The drawing under review shows one solid part. Ordinate dimensions are in mm from its lowest x, y, z. A direction names the side the tool comes from. Give positions to 0.01 mm unless a question says otherwise; leave off trailing zeros. Order: outer loops, then holes, each group sorted by start corner. A loop starts at its lowest first (then second) coordinate and runs counter-clockwise, first axis right, second up. Notation, with made-up numbers: (10, 32) -> (67, 32) arc R24 cw to (67, 71) -> close; hole circle Ø2 at (36.5, 81.5). An arc over 180 degrees is marked (long way). Return JSON: item names as keys, results as strings. Group by question number.
1) Add section B-B (y = 18.5). Give the boundary of the cut face in (x, z), then the cut area to 3 significant figures.
2) Add section C-C (z = 29.5). Give the boundary of the cut face in (x, y).
3) Add section A-A (x = 18). Give the boundary of the cut face in (y, z) (1 decimal), then the cut area to 3 significant figures.
4) Insertion check: P1, Ø2.5, axis at x = 22.5, y = 37, coming from the +Z side; P2, Ø5, axis at y = 38, z = 33.5, coming from the -X side (1 decimal); P3, Ø5, axis at x = 10, y = 24.5, coming from the -Z side. Each pin has a flat end and moves straight along its axis. Give the tip position at first contact, or say it passes through.
5) Add section D-D (x = 36.5). Give the boundary of the cut face in (y, z), then the cut area to 3 significant figures.
6) For the marked faces 1, 2 and 3, list the 3-axis set-ups (+Z, -Z, +X, -X, +Y, -Y) from which the entire face can be reached by the end or side of a thin tool; tool diameter is ignored.
7) To check wall thickness, follow line 1 along Y through (x, z) = (22.5, 13.2); line 2 along Y through (x, z) = (22, 14) (1 decimal); line 3 along Z through (x, y) = (4.5, 22). State the ranges of each line that lie inside material, in increasing order.
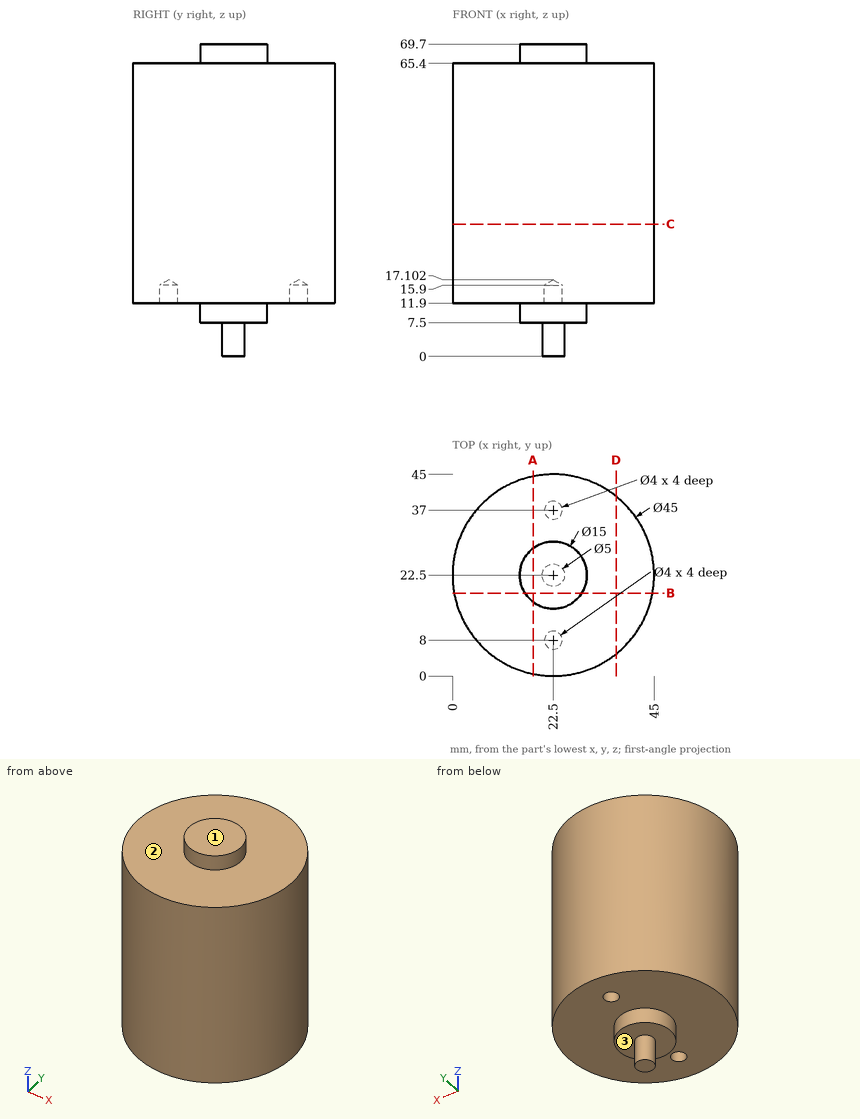
Evaluation:
{
 "1": {"outline": "(0.36, 11.9) -> (16.16, 11.9) -> (16.16, 7.5) -> (28.84, 7.5) -> (28.84, 11.9) -> (44.64, 11.9) -> (44.64, 65.4) -> (28.84, 65.4) -> (28.84, 69.7) -> (16.16, 69.7) -> (16.16, 65.4) -> (0.36, 65.4) -> close", "area": "2,480 mm^2"},
 "2": {"outline": "circle Ø45 at (22.5, 22.5)"},
 "3": {"outline": "(0.5, 11.9) -> (16.5, 11.9) -> (16.5, 7.5) -> (28.5, 7.5) -> (28.5, 11.9) -> (44.5, 11.9) -> (44.5, 65.4) -> (28.5, 65.4) -> (28.5, 69.7) -> (16.5, 69.7) -> (16.5, 65.4) -> (0.5, 65.4) -> close", "area": "2,460 mm^2"},
 "4": {"P1": "z = 65.4", "P2": "x = 4.1", "P3": "z = 11.9"},
 "5": {"outline": "(4.89, 11.9) -> (40.11, 11.9) -> (40.11, 65.4) -> (4.89, 65.4) -> close", "area": "1,880 mm^2"},
 "6": {"face 1": "+Z, +X, -X, +Y, -Y", "face 2": "+Z", "face 3": "-Z"},
 "7": {"line 1": "0 to 6, 10 to 35, 39 to 45", "line 2": "0 to 6.1, 9.9 to 35.1, 38.9 to 45", "line 3": "11.9 to 65.4"}
}
